```python
from build123d import *

# Parameters (mm, degrees)
SALIENTE_EXTRUIR1_DEPTH = 4
CORTAR_EXTRUIR1_DEPTH   = 4


with BuildPart() as part:
    # Croquis1 → Saliente-Extruir1 (new body)
    with BuildSketch(Plane.XY):
        with BuildLine():
            Line((-102.615102368, -94.221952824), (-98.365102368, -94.221952824))
            Line((-98.365102368, -94.221952824), (-98.365102368, -91.221952824))
            Line((-98.365102368, -91.221952824), (-90.365102368, -91.221952824))
            Line((-90.365102368, -91.221952824), (-90.365102368, -94.221952824))
            Line((-90.365102368, -94.221952824), (-86.990102368, -94.221952824))
            ThreePointArc((-86.990102368, -94.221952824), (-84.868782024, -93.343273168), (-83.990102368, -91.221952824))
            Line((-83.990102368, -91.221952824), (-83.990102368, -67.221952824))
            ThreePointArc((-83.990102368, -67.221952824), (-84.868782024, -65.10063248), (-86.990102368, -64.221952824))
            Line((-86.990102368, -64.221952824), (-90.990102368, -64.221952824))
            Line((-90.990102368, -64.221952824), (-90.990102368, -65.721952824))
            Line((-90.990102368, -65.721952824), (-88.490102368, -65.721952824))
            Line((-88.490102368, -65.721952824), (-88.490102368, -68.721952824))
            Line((-88.490102368, -68.721952824), (-97.490102368, -68.721952824))
            Line((-97.490102368, -68.721952824), (-97.490102368, -65.721952824))
            Line((-97.490102368, -65.721952824), (-94.990102368, -65.721952824))
            Line((-94.990102368, -65.721952824), (-94.990102368, -64.221952824))
            Line((-94.990102368, -64.221952824), (-102.615102368, -64.221952824))
            Line((-102.615102368, -64.221952824), (-102.615102368, -60.221952824))
            Line((-102.615102368, -60.221952824), (-105.115102368, -60.221952824))
            Line((-105.115102368, -60.221952824), (-107.615102368, -60.221952824))
            Line((-107.615102368, -60.221952824), (-107.615102368, -64.221952824))
            Line((-107.615102368, -64.221952824), (-115.240102368, -64.221952824))
            Line((-115.240102368, -64.221952824), (-115.240102368, -65.721952824))
            Line((-115.240102368, -65.721952824), (-112.740102368, -65.721952824))
            Line((-112.740102368, -65.721952824), (-112.740102368, -68.721952824))
            Line((-112.740102368, -68.721952824), (-121.740102368, -68.721952824))
            Line((-121.740102368, -68.721952824), (-121.740102368, -65.721952824))
            Line((-121.740102368, -65.721952824), (-119.240102368, -65.721952824))
            Line((-119.240102368, -65.721952824), (-119.240102368, -64.221952824))
            Line((-119.240102368, -64.221952824), (-123.240102368, -64.221952824))
            ThreePointArc((-123.240102368, -64.221952824), (-125.361422711, -65.10063248), (-126.240102368, -67.221952824))
            Line((-126.240102368, -67.221952824), (-126.240102368, -91.221952824))
            ThreePointArc((-126.240102368, -91.221952824), (-125.361422711, -93.343273168), (-123.240102368, -94.221952824))
            Line((-123.240102368, -94.221952824), (-107.615102368, -94.221952824))
            Line((-107.615102368, -94.221952824), (-107.615102368, -98.221952824))
            Line((-107.615102368, -98.221952824), (-105.115102368, -98.221952824))
            Line((-105.115102368, -98.221952824), (-102.615102368, -98.221952824))
            Line((-102.615102368, -98.221952824), (-102.615102368, -94.221952824))
        make_face()
    extrude(amount=SALIENTE_EXTRUIR1_DEPTH)

    # Croquis2 → Cortar-Extruir1 (cut)
    with BuildSketch(Plane.XY.offset(4)):
        with BuildLine():
            Line((-102.365102368, -86.221952824), (-93.990102368, -86.221952824))
            ThreePointArc((-93.990102368, -86.221952824), (-91.868782024, -85.343273168), (-90.990102368, -83.221952824))
            Line((-90.990102368, -83.221952824), (-90.990102368, -76.721952824))
            ThreePointArc((-90.990102368, -76.721952824), (-91.868782024, -74.60063248), (-93.990102368, -73.721952824))
            Line((-93.990102368, -73.721952824), (-116.240102368, -73.721952824))
            ThreePointArc((-116.240102368, -73.721952824), (-118.361422711, -74.60063248), (-119.240102368, -76.721952824))
            Line((-119.240102368, -76.721952824), (-119.240102368, -86.221952824))
            ThreePointArc((-119.240102368, -86.221952824), (-118.361422711, -88.343273168), (-116.240102368, -89.221952824))
            Line((-116.240102368, -89.221952824), (-104.365102368, -89.221952824))
            ThreePointArc((-104.365102368, -89.221952824), (-103.657995587, -88.929059605), (-103.365102368, -88.221952824))
            Line((-103.365102368, -88.221952824), (-103.365102368, -87.221952824))
            ThreePointArc((-103.365102368, -87.221952824), (-103.072209149, -86.514846043), (-102.365102368, -86.221952824))
        make_face()
    extrude(amount=-CORTAR_EXTRUIR1_DEPTH, mode=Mode.SUBTRACT)


solid = part.part
```
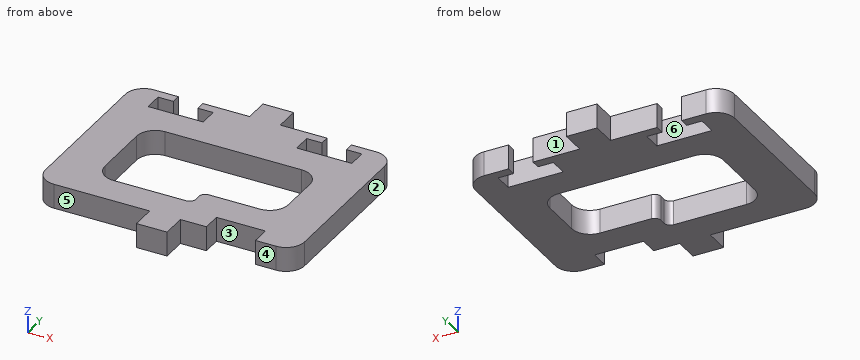
Check sheet for the modelled part. Datum: model origin and axes. Units: mm. Face numbers are marked on the shaded views. A direction names the side the tool comes from. Give positions to 0.01 mm unless a question says otherwise; leave off trailing zeros. Loops run counter-clockwise (first coordinate to the right, second up) from the corner with the lowest first, then second, coordinate; pieces in that order, holes last. Notation, with made-up numbers: (-36, 45.25) - (-5, 45.25) arc R12 cw to (-5, 64.25) - close; hole circle Ø4 at (78.25, 41.25). An arc over 180 degrees is marked (long way). One line per question, with ' | ' between items. Start each with the question number.
1. Cross-section at C-C, the plane x = -96. Enter the section's corners in (y, z).
2. Set-up check for the marked faces 4, 5 and 6: record each of +Z, -Z, +X, -X, +Y, -Y from which the full face is reachable in a straight line by a thin tool's end or side.
3. Draft check along X on the marked faces 1, 2 and 3. Enter one of: released by +X, released by -X, zero draft, split by the parting line, or undercut.
4. Cross-section at A-A, the plane x = -120. Enter the section's corners in (y, z), plus the area to 3 significant figures.
5. Cross-section at D-D, the plane y = -95. Enter the section's corners in (x, z).
6. Gauge pin test, flat ends, axial feed: pin 1 Ø2 at (x, z) = (-122, 1) entering from +Y; pin 2 Ø0.8 at (x, z) = (-96.5, 2) entering from -Y; pin 3 Ø1.2 at (y, z) = (-65, 2) entering from -X. Record the tip position at first contact, or that the pin passes through.
7. Material ranges on line 1 along X through (y, z) = (-67, 3.65); line 2 along Y through (x, z) = (-97, 2.4); line 3 along Y through (x, z) = (-113.5, 1.1), recorded low to high. Write a range as [from, to].
8. Cross-section at B-B, the plane y = -81. Enter the section's corners in (x, z).
Check result:
1) outline: (-91.22, 0) - (-86.22, 0) - (-86.22, 4) - (-91.22, 4) - close; (-73.72, 0) - (-68.72, 0) - (-68.72, 4) - (-73.72, 4) - close; (-65.72, 0) - (-64.22, 0) - (-64.22, 4) - (-65.72, 4) - close
2) face 4: +Z, -Z, +X, -Y | face 5: +Z, -Z, -X, -Y | face 6: +Z, -Z
3) face 1: zero draft | face 2: released by +X | face 3: undercut
4) outline: (-94.22, 0) - (-68.72, 0) - (-68.72, 4) - (-94.22, 4) - close; (-65.72, 0) - (-64.22, 0) - (-64.22, 4) - (-65.72, 4) - close | area: 108 mm2
5) outline: (-107.62, 0) - (-102.62, 0) - (-102.62, 4) - (-107.62, 4) - close
6) pin 1: stops at y = -64.22 | pin 2: stops at y = -91.22 | pin 3: stops at x = -125.76
7) line 1: x = [-126.23, -121.74], [-112.74, -97.49], [-88.49, -84] | line 2: y = [-91.22, -86.22], [-73.72, -68.72], [-65.72, -64.22] | line 3: y = [-94.22, -89.22], [-73.72, -68.72], [-65.72, -64.22]
8) outline: (-126.24, 0) - (-119.24, 0) - (-119.24, 4) - (-126.24, 4) - close; (-90.99, 0) - (-83.99, 0) - (-83.99, 4) - (-90.99, 4) - close
